Source: CAD feature listing. Evaluate the final solid. Frame: model axes, mm. A direction names the side the tool comes from. Give positions to 0.01 mm unless a question says otherwise; leave off trailing zeros. Order: outer loops, then holes, each group sorted by start corner. A loop starts at its lowest first (then second) coordinate and runs counter-clockwise, first axis right, second up.
1) Material intervals for line 1 (Y direction, x = 0.05, z = 18); line 2 (X direction, y = -1.25, z = 93); line 3 (X direction, y = -1.5, z = 81), sorted ascending.
2) First-contact query: P1, Ø0.9, axis at y = -2, z = 91, coming from the -X side; P2, Ø0.6, axis at x = 2, z = 92.5, coming from the +Y side; P3, Ø1, axis at y = -1, z = 55.5, coming from the +X side. Flat tips, straight axial feed; report the tip coordinate or a pass-through.
3) Access query for faces 1 (the face through (-1.514, -0.026, 7.605)), 2 (the face through (-1, 3, 91)), 3 (the face through (1.486, 0.026, 7.395)), 4 (the face through (1, 3, 91)), 5 (the face through (1, -2, 91)). Directions: +Z, -Z, +X, -X, +Y, -Y. A direction counts if a zero-diameter tool reaches every point of the face in a straight line with its end or side. Return the directions, or none.
4) Draft query along Z for faces 6 (the face through (2.31, -0.96, 53.71)), 7 (the face through (-1, -2, 91)), 8 (the face through (0.02, -1.74, 7.4)). Return one class per face: released by +Z, released by -Z, zero draft, split by the parting line, or undercut.
5) Section A-A, the plane y = 0. Return loops of the section in (x, z).
6) Section B-B, the plane z = 64. Return loops of the section in (x, y), plus the area to 3 significant figures.
```python
from build123d import *

# Parameters (mm, degrees)
SKETCH1_R           = 2.5
BOSS_EXTRUDE1_DEPTH = 100
CUT_EXTRUDE1_DEPTH  = 5
BOSS_EXTRUDE2_DEPTH = 1
CUT_EXTRUDE2_DEPTH  = 6
CUT_EXTRUDE3_DEPTH  = 2.5


with BuildPart() as part:
    # Sketch1 → Boss-Extrude1 (new body)
    with BuildSketch(Plane.XY):
        Circle(SKETCH1_R)
    extrude(amount=BOSS_EXTRUDE1_DEPTH)

    # Sketch2 → Cut-Extrude1 (cut, symmetric)
    with BuildSketch(Plane(origin=(0, 0, 0), x_dir=(0, 0, -1), z_dir=(1, 0, 0))):
        with BuildLine():
            Line((-94, 4), (-88, 4))
            ThreePointArc((-88, 4), (-87.292893219, 3.707106781), (-87, 3))
            Line((-87, 3), (-87, 2))
            ThreePointArc((-87, 2), (-87.292893219, 1.292893219), (-88, 1))
            Line((-88, 1), (-94, 1))
            ThreePointArc((-94, 1), (-94.707106781, 1.292893219), (-95, 2))
            Line((-95, 2), (-95, 3))
            ThreePointArc((-95, 3), (-94.707106781, 3.707106781), (-94, 4))
        make_face()
        with BuildLine():
            Line((-87, -3), (-87, -2))
            ThreePointArc((-87, -2), (-87.292893219, -1.292893219), (-88, -1))
            Line((-88, -1), (-94, -1))
            ThreePointArc((-94, -1), (-94.707106781, -1.292893219), (-95, -2))
            Line((-95, -2), (-95, -3))
            ThreePointArc((-95, -3), (-94.707106781, -3.707106781), (-94, -4))
            Line((-94, -4), (-88, -4))
            ThreePointArc((-88, -4), (-87.292893219, -3.707106781), (-87, -3))
        make_face()
    extrude(amount=CUT_EXTRUDE1_DEPTH, both=True, mode=Mode.SUBTRACT)

    # Sketch2<2> → Boss-Extrude2 (add, symmetric)
    with BuildSketch(Plane(origin=(0, 0, 0), x_dir=(0, 0, -1), z_dir=(1, 0, 0))):
        with BuildLine():
            Line((-94, 4), (-88, 4))
            ThreePointArc((-88, 4), (-87.292893219, 3.707106781), (-87, 3))
            Line((-87, 3), (-87, 2))
            ThreePointArc((-87, 2), (-87.292893219, 1.292893219), (-88, 1))
            Line((-88, 1), (-94, 1))
            ThreePointArc((-94, 1), (-94.707106781, 1.292893219), (-95, 2))
            Line((-95, 2), (-95, 3))
            ThreePointArc((-95, 3), (-94.707106781, 3.707106781), (-94, 4))
        make_face()
        with BuildLine():
            Line((-87, -3), (-87, -2))
            ThreePointArc((-87, -2), (-87.292893219, -1.292893219), (-88, -1))
            Line((-88, -1), (-94, -1))
            ThreePointArc((-94, -1), (-94.707106781, -1.292893219), (-95, -2))
            Line((-95, -2), (-95, -3))
            ThreePointArc((-95, -3), (-94.707106781, -3.707106781), (-94, -4))
            Line((-94, -4), (-88, -4))
            ThreePointArc((-88, -4), (-87.292893219, -3.707106781), (-87, -3))
        make_face()
    extrude(amount=BOSS_EXTRUDE2_DEPTH, both=True)

    # Sketch3 → Cut-Extrude2 (cut, symmetric)
    with BuildSketch(Plane(origin=(0, 0, 0), x_dir=(0, 0, -1), z_dir=(1, 0, 0))):
        Polygon((-15, 2.5), (0, 1), (0, 2.5), align=None)
        Polygon((0, -2.5), (0, -1), (-15, -2.5), align=None)
    extrude(amount=CUT_EXTRUDE2_DEPTH, both=True, mode=Mode.SUBTRACT)

    # Sketch4 → Cut-Extrude3 (cut, symmetric)
    with BuildSketch(Plane(origin=(0, 0, 0), x_dir=(1, 0, 0), z_dir=(0, 1, 0))):
        Polygon((-2.5, -15), (-0.5, 0), (-2.5, 0), align=None)
        Polygon((2.5, 0), (0.5, 0), (2.5, -15), align=None)
    extrude(amount=CUT_EXTRUDE3_DEPTH, both=True, mode=Mode.SUBTRACT)


solid = part.part
```
From the geometry:
1. line 1: y = -2.5 to 2.5
1. line 2: x = -1 to 1
1. line 3: x = -2 to 2
2. P1: stops at x = -1
2. P2: stops at y = 1
2. P3: stops at x = 2.45
3. face 1: -Z, -X, +Y, -Y
3. face 2: -X, +Y
3. face 3: -Z, +X, +Y, -Y
3. face 4: +X, +Y
3. face 5: +X, -Y
4. face 6: zero draft
4. face 7: undercut
4. face 8: released by -Z
5. outline: (-2.5, 15) - (-0.5, 0) - (0.5, 0) - (2.5, 15) - (2.5, 100) - (-2.5, 100) - close
6. outline: circle Ø5 at (0, 0)
6. area: 19.6 mm2
